from build123d import *

# Parameters (mm, degrees)
F0_R      = 90
F0_R_2    = 8
F1_DEPTH  = 11
F2_R      = 50
F3_DEPTH  = 310
F4_R      = 44
F5_DEPTH  = 190
F6_R      = 35
F7_DEPTH  = 350
F8_SIZE   = 5.99999
F10_R     = 50
F11_DEPTH = 8
F12_SIZE  = 5.99999


# Not quite as in the source:
# - a fillet or chamfer is up to 0.001 mm smaller than in the source, because OpenCascade refuses the exact size


with BuildPart() as f1:
    # F0 (on Front) → F1 (new body)
    with BuildSketch(Plane.XZ):
        Circle(F0_R)
        with Locations((0, 77.5)):
            Circle(F0_R_2, mode=Mode.SUBTRACT)
    extrude(amount=F1_DEPTH)

    # F2 (on face) → F3 (join)
    with BuildSketch(Plane.XZ.offset(11)):
        Circle(F2_R)
    extrude(amount=F3_DEPTH)

    # F4 (on face) → F5 (join)
    with BuildSketch(Plane.XZ.offset(321)):
        Circle(F4_R)
    extrude(amount=F5_DEPTH)

    # F6 (on face) → F7 (cut)
    with BuildSketch(Plane.XZ.offset(511)):
        Circle(F6_R)
    extrude(amount=-F7_DEPTH, mode=Mode.SUBTRACT)

    # F8 (size 6 in the source; OpenCascade refuses exactly that, so slightly less here)
    f8_edges = [f1.edges().sort_by_distance(p)[0] for p in [
        (-50, -321, 0),
    ]]
    chamfer(f8_edges, length=F8_SIZE)

    # F10 (on offset) → F11 (join)
    with BuildSketch(Plane.XZ.offset(371)):
        Circle(F10_R)
    extrude(amount=-F11_DEPTH)

    # F12 (size 6 in the source; OpenCascade refuses exactly that, so slightly less here)
    f12_edges = [f1.edges().sort_by_distance(p)[0] for p in [
        (-50, -363, 0),
    ]]
    chamfer(f12_edges, length=F12_SIZE)


solid = f1.part
Read the model definition and answer for the solid it produces. Units are mm, in the model's axes. A direction names the side the tool comes from. Coordinates: 2 decimals unless noted, no trailing zeros. Loops run counter-clockwise (first coordinate to the right, second up) from the corner with the lowest first, then second, coordinate; pieces in that order, holes last. Notation, with made-up numbers: (30.5, 79.25) - (51.5, 79.25) arc R23 cw to (51.5, 98.25) - close; hole circle Ø2 at (77.5, -16.75). An arc over 180 degrees is marked (long way). Answer in a Markdown table with one row per item.
Q1. For faces 1 (the cylindrical face through (47.69, -370.01, 15.02)), 2 (the flat face through (0, -161, 0)), 3 (the cylindrical face through (-1.041, -5.423, 85.432)), determine the directions among +Z, -Z, +X, -X, +Y, -Y from which every point of the face is accessible in a straight line to the end or side of a thin tool.
Here are the results:
| item | result |
|---|---|
| face 1 | -Y |
| face 2 | none |
| face 3 | +Y, -Y |
Q2. Straight lines are drawn through the part: line 1 along Y through (x, z) = (15.5, 22.5); line 2 along Z through (x, y) = (0, -5); line 3 along Z through (x, y) = (0, -459.5). For each, find the intervals that lie inside material, in ascending order. Write a range as [from, to].
Here are the results:
| item | result |
|---|---|
| line 1 | y = [-371, -363], [-161, 0] |
| line 2 | z = [-90, 69.5], [85.5, 90] |
| line 3 | z = [-44, -35], [35, 44] |
Q3. The mould has two halves that part along X. Classify faces 4 (the cylindrical face through (-9.538, -341.706, -42.954)), 5 (the flat face through (-0.2, -371, -44.2)), 6 (the flat face through (0, -363, 0)): pulls with the +X half, pulls with the -X half, needs draft (parallel to the pull), parting line crosses it, or undercut.
Here are the results:
| item | result |
|---|---|
| face 4 | parting line crosses it |
| face 5 | needs draft |
| face 6 | undercut |
Q4. Find section D-D on z = 77.5. Write down the section's boundary in (x, y).
Here are the results:
| item | result |
|---|---|
| outline | (-45.76, -11) - (-8, -11) - (-8, 0) - (-45.76, 0) - close; (8, -11) - (45.76, -11) - (45.76, 0) - (8, 0) - close |
Q5. Find section C-C on x = 0. Count the separate pieces of the cut face and the enclosed holes in it, plus the area to 3 significant figures.
Here are the results:
| item | result |
|---|---|
| separate pieces | 2 |
| enclosed holes | 1 |
| area | 25,600 mm^2 |
Q6. Given P1, Ø9.5, axis at x = 0, z = 77.5, coming from the -Y side; P2, Ø6, axis at y = -297, z = 20.5, coming from the +X side; P3, Ø3, axis at x = -32, z = 14, coming from the -Y side; P4, Ø1, axis at y = -313.5, z = -37.5, coming from the +X side, each flat-ended and moving along its own axis, determine where each tip first touches the part or whether it passes through.
Here are the results:
| item | result |
|---|---|
| P1 | passes through |
| P2 | stops at x = 46.84 |
| P3 | stops at y = -511 |
| P4 | stops at x = 33.63 |
Q7. Find section B-B on y = -293.5. Write down the section's boundary in (x, z).
Here are the results:
| item | result |
|---|---|
| outline | circle Ø100 at (0, 0); hole circle Ø70 at (0, 0) |
